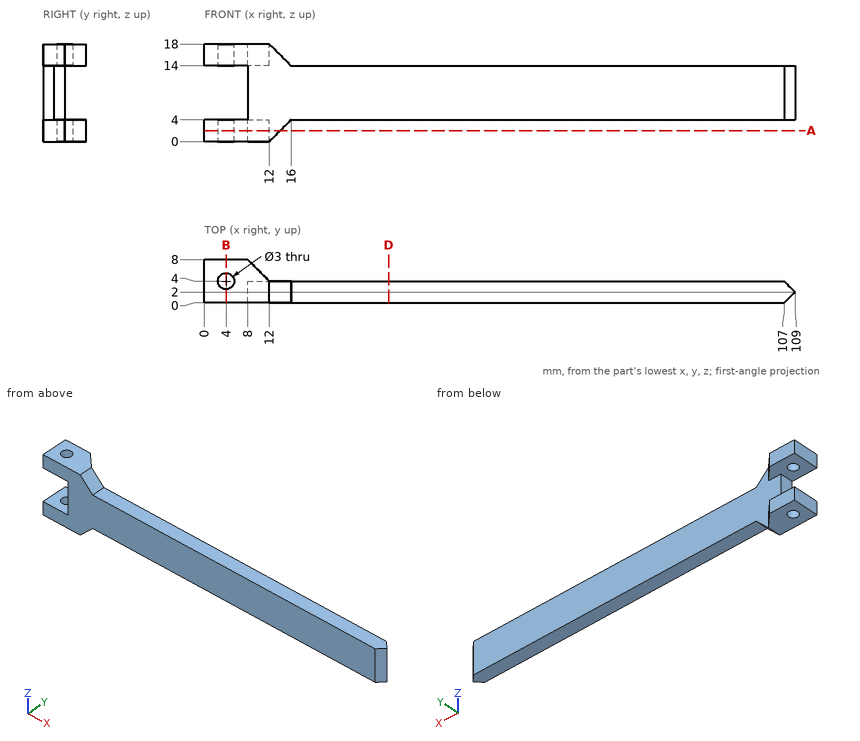
Check sheet for the drawn part. Datum: minimum x, y, z corner. Units: mm. Coordinates: 2 decimals unless noted, no trailing zeros. Write each loop counter-clockwise with the first axis right and the second up, starting at its lowest first coordinate (ties: lowest second). Pieces come first, ordered by that corner, then holes. Notation, with made-up numbers: M 38,-35 L 78,-35 A23 ccw 78,-16 Z; hole C -24.5,81.25 d9. An arc over 180 degrees is marked long. One line per item, written item: value.
Item 1: Section check B-B, the plane x = 4. Record the boundary of the cut face in (y, z), plus the area to 3 significant figures.
Check sheet entries:
outline: M 0,0 L 2.5,0 L 2.5,4 L 0,4 Z; M 0,14 L 2.5,14 L 2.5,18 L 0,18 Z; M 5.5,0 L 8,0 L 8,4 L 5.5,4 Z; M 5.5,14 L 8,14 L 8,18 L 5.5,18 Z
area: 40.0 mm^2
Item 2: Section check D-D, the plane x = 34. Record the boundary of the cut face in (y, z).
Check sheet entries:
outline: M 0,4 L 4,4 L 4,14 L 0,14 Z
Item 3: Gauge pin test, flat ends, axial feed: pin 1 Ø4.5 at (x, y) = (43, 2.5) entering from -Z; pin 2 Ø2 at (x, z) = (46, 7) entering from +Y; pin 3 Ø2 at (x, y) = (77.5, 2) entering from +Z. Record the tip position at first contact, or that the pin passes through.
Check sheet entries:
pin 1: stops at z = 4
pin 2: stops at y = 4
pin 3: stops at z = 14
Item 4: Section check A-A, the plane z = 2. Record the boundary of the cut face in (x, y).
Check sheet entries:
outline: M 0,0 L 14,0 L 14,4 L 12,4 L 8,8 L 0,8 Z; hole C 4,4 d3
Item 5: Scan lines: line 1 along Y through (x, z) = (4, 3.2); line 2 along Z through (x, y) = (6, 5.25); line 3 along Z through (x, y) = (68, 3.75). Record each from-to range of solid material in increasing order.
Check sheet entries:
line 1: y = 0 to 2.5, 5.5 to 8
line 2: z = 0 to 4, 14 to 18
line 3: z = 4 to 14
